```python
from build123d import *

# Parameters (mm, degrees)
F1_DEPTH = 12.7
F2_W     = 139.7
F2_H     = 68.58
F3_DEPTH = 8.89
F4_R     = 5.08
F5_R     = 17
F6_DEPTH = 95
F7_R     = 5.08


with BuildPart() as f1:
    # F0 (on Right) → F1 (new body)
    with BuildSketch(Plane.YZ):
        with BuildLine():
            Line((74.93, 43.18), (-74.93, 43.18))
            ThreePointArc((-74.93, 43.18), (-79.420128, 41.320128), (-81.28, 36.83))
            Line((-81.28, 36.83), (-81.28, -36.83))
            ThreePointArc((-81.28, -36.83), (-79.420128, -41.320128), (-74.93, -43.18))
            Line((-74.93, -43.18), (74.93, -43.18))
            ThreePointArc((74.93, -43.18), (79.420128, -41.320128), (81.28, -36.83))
            Line((81.28, -36.83), (81.28, 36.83))
            ThreePointArc((81.28, 36.83), (79.420128, 41.320128), (74.93, 43.18))
        make_face()
    extrude(amount=F1_DEPTH)

    # F2 (on face) → F3 (cut)
    with BuildSketch(Plane.YZ.offset(12.7)):
        Rectangle(F2_W, F2_H)
    extrude(amount=-F3_DEPTH, mode=Mode.SUBTRACT)

    # F4
    f4_edges = [f1.edges().sort_by_distance(p)[0] for p in [
        (12.7, 81.28, 0),
        (12.7, 0, 43.18),
        (12.7, -81.28, 0),
        (12.7, 0, -43.18),
    ]]
    fillet(f4_edges, radius=F4_R)

    # F5 (on face) → F6 (join)
    with BuildSketch(Plane(origin=(0, 0, 0), x_dir=(0, -1, 0), z_dir=(-1, 0, 0))):
        with Locations((-64.28, 0)):
            Circle(F5_R)
        with Locations((64.28, 0)):
            Circle(F5_R)
    extrude(amount=F6_DEPTH)

    # F7
    f7_edges = [f1.edges().sort_by_distance(p)[0] for p in [
        (-95, -47.28, 0),
        (-95, 81.28, 0),
    ]]
    fillet(f7_edges, radius=F7_R)


solid = f1.part
```
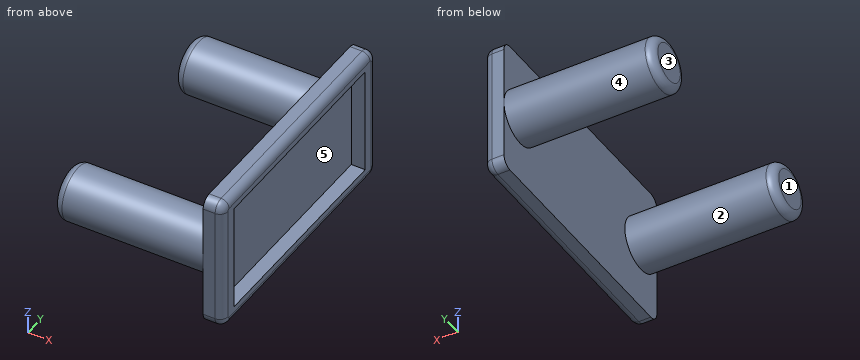
Can you work these out from the model? Positions are in its coordinate system, mm. Face numbers are marked on the shaded views. A direction names the side the tool comes from. Coordinates: 2 decimals unless noted, no trailing zeros. Order: outer loops, then holes, each group sorted by start corner. A loop starts at its lowest first (then second) coordinate and runs counter-clockwise, first axis right, second up.
1. If we section it at C-C (x = -51.5): Please give me the cut outline in (y, z).
2. If we section it at D-D (y = 9): Please give me the cut outline in (x, z), then the cut area to 3 significant figures.
3. I need wall thicknesses on line 1 (Y direction, x = 8, z = 21.5); line 2 (X direction, y = 25, z = 1.5); line 3 (Y direction, x = -76, z = -15.5). Which ranges of each line are inside material? Lowest first, please.
4. If we section it at B-B (z = 19.5): Please give me the cut outline in (x, y).
5. For the marked faces 3, 4 and 5, which set-ups out of +Z, -Z, +X, -X, +Y, -Y let a thin tool reach every point of the face, with its end or its side?
6. I'm going to push flat-ended pins straight in: pin 1 (10 mm diameter, centred on y = -4, z = -34, fed in from -X); pin 2 (5 mm diameter, centred on x = -18.5, y = -54.5, fed in from -Z); pin 3 (4 mm diameter, centred on x = -81, y = -56, fed in from -Z). Where does each tip first touch, or does it pass through?
7. Thinking about a two-plate mould opening in Y: for the marked faces 1 and 2, which applies, +Y half, -Y half, draft (parallel to the pull), parting line (faces both ways), or undercut?
8. If we section it at A-A (y = 64.28): Please give me the cut outline in (x, z).
Entries:
1. outline: circle Ø34 at (-64.28, 0); circle Ø34 at (64.28, 0)
2. outline: (0, -43.18) - (7.62, -43.18) arc R5.08 ccw to (12.7, -38.1) - (12.7, -34.29) - (3.81, -34.29) - (3.81, 34.29) - (12.7, 34.29) - (12.7, 38.1) arc R5.08 ccw to (7.62, 43.18) - (0, 43.18) - close
2. area: 476 mm2
3. line 1: y = -81.27 to -69.85, 69.85 to 81.27
3. line 2: x = 0 to 3.81
3. line 3: y = -71.26 to -57.3, 57.3 to 71.26
4. outline: (0, -81.28) - (7.62, -81.28) arc R5.08 ccw to (12.7, -76.2) - (12.7, -69.85) - (3.81, -69.85) - (3.81, 69.85) - (12.7, 69.85) - (12.7, 76.2) arc R5.08 ccw to (7.62, 81.28) - (0, 81.28) - close
5. face 3: +Z, -Z, -X, +Y, -Y
5. face 4: -X
5. face 5: +X
6. pin 1: stops at x = 0
6. pin 2: stops at z = -15.36
6. pin 3: stops at z = -15.8
7. face 1: draft
7. face 2: undercut
8. outline: (-95, -11.92) arc R5.08 ccw to (-89.92, -17) - (0, -17) - (0, -43.18) - (7.62, -43.18) arc R5.08 ccw to (12.7, -38.1) - (12.7, -34.29) - (3.81, -34.29) - (3.81, 34.29) - (12.7, 34.29) - (12.7, 38.1) arc R5.08 ccw to (7.62, 43.18) - (0, 43.18) - (0, 17) - (-89.92, 17) arc R5.08 ccw to (-95, 11.92) - close
